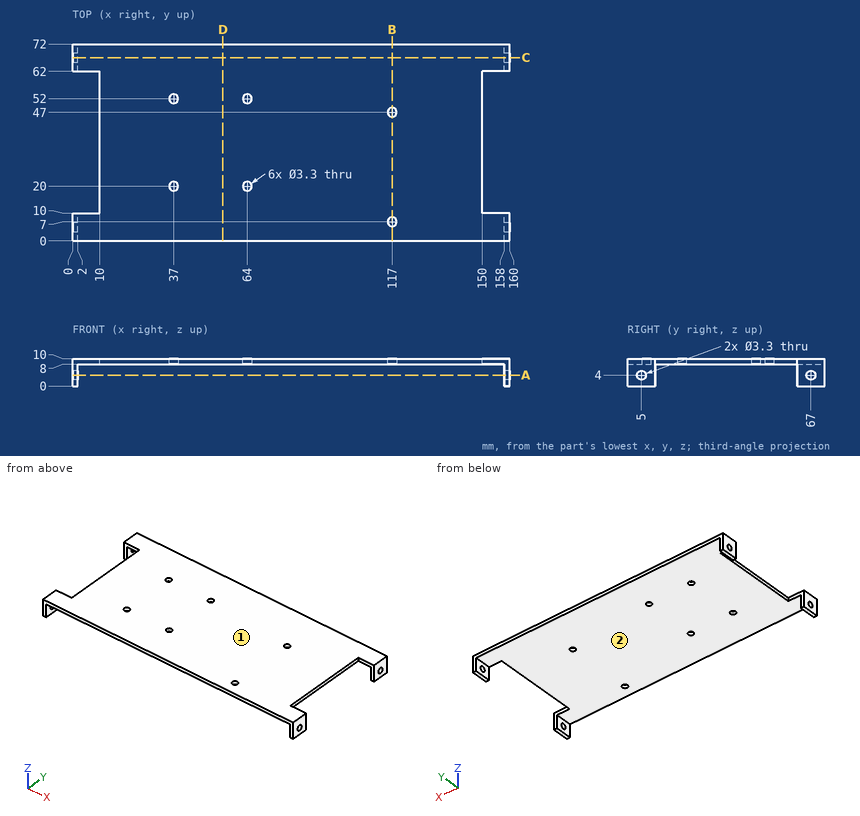
Geometry check sheet. Reference: drawing and pictorial views, mm from the part's lowest x, y, z. A direction names the side the tool comes from. Round coordinates to 2 decimals unless told otherwise and drop trailing zeros. Loops run counter-clockwise (first coordinate to the right, second up) from the corner with the lowest first, then second, coordinate; pieces in that order, holes last. Notation, with made-up numbers: (12.5, 40) - (36.5, 40) arc R27 ccw to (36.5, 58) - close; hole circle Ø3 at (67.5, -1). An arc over 180 degrees is marked (long way). Use a Markdown table: item, result.
Q1. Cross-section at D-D on x = 55. Record the cut outline in (y, z).
Solutions:
| item | result |
|---|---|
| outline | (0, 8) - (72, 8) - (72, 10) - (0, 10) - close |
Q2. Go/stop test with flat-tipped pins: P1, Ø3, axis at x = 141.5, y = 55, coming from the -Z side; P2, Ø6, axis at y = 45, z = 7.5, coming from the +X side; P3, Ø5, axis at y = 14, z = 1.5, coming from the +X side; P4, Ø1, axis at y = 34, z = 9.5, coming from the -X side. Record where each tip stops, or that it passes through.
Solutions:
| item | result |
|---|---|
| P1 | stops at z = 8 |
| P2 | stops at x = 150 |
| P3 | passes through |
| P4 | stops at x = 10 |
Q3. Cross-section at B-B on x = 117. Record the cut outline in (y, z), plus the area to 3 significant figures.
Solutions:
| item | result |
|---|---|
| outline | (0, 8) - (5.35, 8) - (5.35, 10) - (0, 10) - close; (8.65, 8) - (45.35, 8) - (45.35, 10) - (8.65, 10) - close; (48.65, 8) - (72, 8) - (72, 10) - (48.65, 10) - close |
| area | 131 mm2 |
Q4. Access from +Z, -Z, +X, -X, +Y, -Y to the whole of each face (thin tool, end or side, straight path). Record for the marked faces 1 and 2.
Solutions:
| item | result |
|---|---|
| face 1 | +Z, +X, -X, +Y, -Y |
| face 2 | -Z, +Y, -Y |
Q5. Material ranges on line 1 (Y direction, x = 64, z = 9.35); line 2 (Y direction, x = 117, z = 9.05); line 3 (Z direction, x = 1.15, y = 67), recorded low to high.
Solutions:
| item | result |
|---|---|
| line 1 | y = 0 to 18.35, 21.65 to 50.35, 53.65 to 72 |
| line 2 | y = 0 to 5.35, 8.65 to 45.35, 48.65 to 72 |
| line 3 | z = 0 to 2.35, 5.65 to 10 |
Q6. Cross-section at A-A on z = 4. State how many separate pieces and enclosed holes the cut face has, plus the area to 3 significant figures.
Solutions:
| item | result |
|---|---|
| separate pieces | 8 |
| enclosed holes | 0 |
| area | 53.6 mm2 |
Q7. Cross-section at C-C on y = 67. Record the cut outline in (x, z), plus the area to 3 significant figures.
Solutions:
| item | result |
|---|---|
| outline | (0, 0) - (2, 0) - (2, 2.35) - (0, 2.35) - close; (0, 5.65) - (2, 5.65) - (2, 8) - (158, 8) - (158, 5.65) - (160, 5.65) - (160, 10) - (0, 10) - close; (158, 0) - (160, 0) - (160, 2.35) - (158, 2.35) - close |
| area | 339 mm2 |
